Check sheet for the modelled part. Datum: model origin and axes. Units: mm. Face numbers are marked on the shaded views. A direction names the side the tool comes from. Round coordinates to 2 decimals unless told otherwise and drop trailing zeros. Order: outer loops, then holes, each group sorted by start corner. A loop starts at its lowest first (then second) coordinate and runs counter-clockwise, first axis right, second up. Notation, with made-up numbers: (-24, -28) -> (-16, -28) arc R30 ccw to (-16, 4) -> close; hole circle Ø4 at (48, -20.5). An arc over 180 degrees is marked (long way). Answer in a Markdown table with one row per item. Add a question column.
1. Draft check along Y on the marked faces 3, 4 and 5. Enter one of: +Y half, -Y half, draft (parallel to the pull), parting line (faces both ways), or undercut.
2. Sectioned sample at C-C, the plane x = -19.5. Record the boundary of the cut face in (y, z) (3 decimals).
3. Access from +Z, -Z, +X, -X, +Y, -Y to the whole of each face (thin tool, end or side, straight path). Record for the marked faces 1 and 2.
4. Sectioned sample at D-D, the plane z = 14.25. Record the boundary of the cut face in (x, y).
5. Depth check by flat-ended pin: P1, Ø1.5, axis at x = 21.5, z = 9, coming from the -Y side; P2, Ø4, axis at x = -46.5, z = 5.5, coming from the -Y side; P3, Ø3, axis at x = 17, y = 11, coming from the +Z side (3 decimals). Enter the tip coordinate at first touch or a pass-through.
6. Sectioned sample at B-B, the plane y = 0.5. Record the boundary of the cut face in (x, z) (3 decimals), then the cut area to 3 significant figures.
7. Material ranges on L1, parallel to X at y = -44, z = 17.25; L2, parallel to Y at x = -58, z = 11.75; L3, parallel to Z at x = -33, y = -11 (3 decimals), recorded low to high. Write a range as from..to.
Autodesk Inventor part; units mm, degrees
ref_plane "YZ Plane" through (0, 0, 0) normal (1, 0, 0) x (0, 1, 0)
ref_plane "XZ Plane" through (0, 0, 0) normal (0, 1, 0) x (-1, 0, 0)
ref_plane "XY Plane" through (0, 0, 0) normal (0, 0, 1) x (1, 0, 0)
sketch "Sketch1" plane through (0, 0, 0) normal (0, 0, 1) x (1, 0, 0)
  line L0 (-65.5382, -61.3942) -> (80.107, 40.5877)
  line L1 (80.107, 40.5877) -> (65.5382, 61.3942)
  line L2 (65.5382, 61.3942) -> (-80.107, -40.5877)
  line L3 (-80.107, -40.5877) -> (-65.5382, -61.3942)
  line L4 (-65.5382, -61.3942) -> (65.5382, 61.3942) construction
  line L5 (80.107, 40.5877) -> (-80.107, -40.5877) construction
  line L6 (-65.5382, -61.3942) -> (112.2618, -61.3942) construction
  point P0 (0, 0)
  dimension "d0" = 177.8
  dimension "d1" = 35
  dimension "d2" = 25.4
extrude "Extrusion1" add sketch "Sketch1" along normal blind 9.525
sketch "Sketch2" plane through (0, 0, 9.525) normal (0, 0, 1) x (1, 0, 0)
  point P0 (0, 0)
fillet "Fillet1" radius 12.7 4 edges at (65.5382, 61.3942, 4.7625) (80.107, 40.5877, 4.7625) (-65.5382, -61.3942, 4.7625) (-80.107, -40.5877, 4.7625)
sketch "Sketch3" plane through (0, 0, 9.525) normal (0, 0, 1) x (1, 0, 0)
  arc A0 (-69.7038, -33.3033) -> (-55.135, -54.1098) centre (-62.4194, -43.7065) ccw construction
  line L0 (-54.5275, -43.0212) -> (-57.88, -50.1984)
  line L1 (-57.88, -50.1984) -> (-65.7718, -50.8837)
  line L2 (-65.7718, -50.8837) -> (-70.3112, -44.3918)
  line L3 (-70.3112, -44.3918) -> (-66.9588, -37.2146)
  line L4 (-66.9588, -37.2146) -> (-59.0669, -36.5293)
  line L5 (-59.0669, -36.5293) -> (-54.5275, -43.0212)
  point P0 (0, 0)
sketch "Sketch4" plane through (0, 0, 9.525) normal (0, 0, 1) x (1, 0, 0)
  arc A0 (-69.7038, -33.3033) -> (-55.135, -54.1098) centre (-62.4194, -43.7065) ccw
  line L0 (55.135, 54.1098) -> (-69.7038, -33.3033)
  circle A1 centre (-62.4194, -43.7065) radius 12.7
  point P0 (0, 0)
  point P1 (-55.135, -54.1098)
extrude "Extrusion2" add sketch "Sketch4" along normal blind 9.525
extrude "Extrusion3" cut sketch "Sketch3" against normal mid plane 25.4
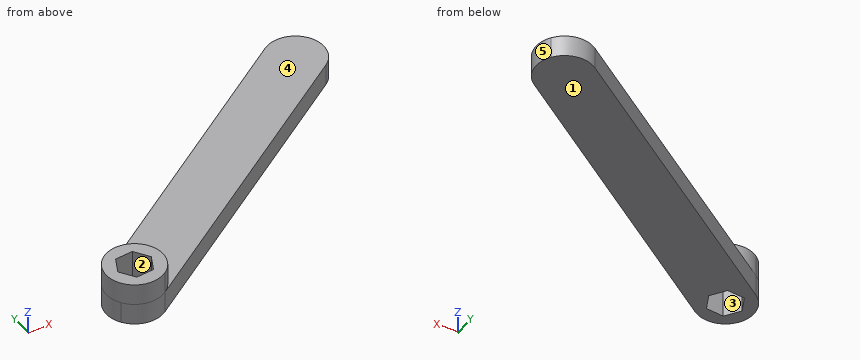
Answer key:
| question | item | result |
|---|---|---|
| 1 | face 3 | undercut |
| 1 | face 4 | draft |
| 1 | face 5 | parting line |
| 2 | outline | (-29.158, 0) -> (1.85, 0) -> (1.85, 9.525) -> (-29.158, 9.525) -> close |
| 3 | face 1 | -Z, +X, -X, +Y, -Y |
| 3 | face 2 | +Z, -Z |
| 4 | outline | (-69.7, -33.3) arc R12.7 ccw to (-55.13, -54.11) arc R12.7 ccw to start; hole (-70.31, -44.39) -> (-65.77, -50.88) -> (-57.88, -50.2) -> (-54.53, -43.02) -> (-59.07, -36.53) -> (-66.96, -37.21) -> close |
| 5 | P1 | stops at y = -0.97 |
| 5 | P2 | stops at y = -49.46 |
| 5 | P3 | stops at z = 9.525 |
| 6 | outline | (-21.428, 0) -> (22.856, 0) -> (22.856, 9.525) -> (-21.428, 9.525) -> close |
| 6 | area | 422 mm² |
| 7 | L1 | x = -75.12..-70.13, -54.98..-49.72 |
| 7 | L2 | y = -55.61..-50.21, -38.06..-31.8 |
| 7 | L3 | z = 0..9.525 |
